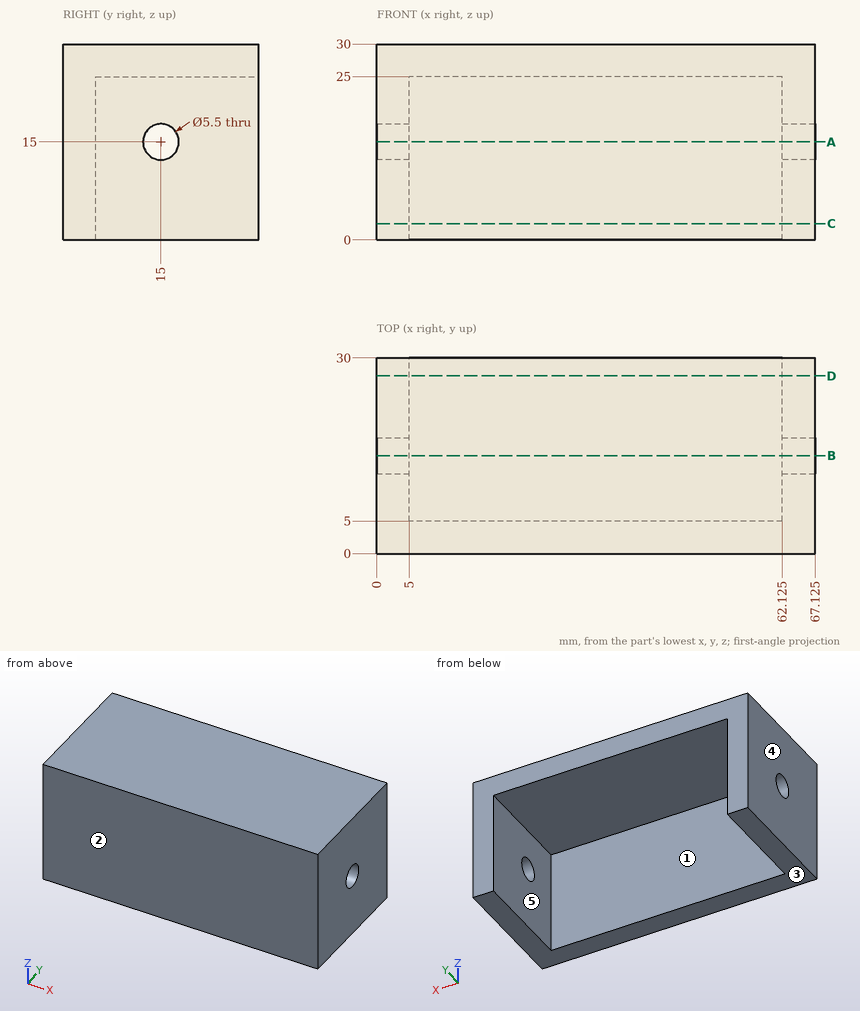
Design review of the part shown in the three views and the two pictorial views. Dimensions are in mm from the part's minimum x, y and z. A direction names the side the tool comes from. Round coordinates to 2 decimals unless told otherwise and drop trailing zeros. Order: outer loops, then holes, each group sorted by start corner. A loop starts at its lowest first (then second) coordinate and runs counter-clockwise, first axis right, second up.
(1) Mouldability with a two-part tool opening along X and no side actions: class the marked faces 3, 4 and 5 as released by +X, released by -X, zero draft, split by the parting line, or undercut.
Working result:
face 3: zero draft
face 4: released by -X
face 5: undercut
(2) For P1, Ø3, axis at x = 58.5, z = 15, coming from the +Y side; P2, Ø12.5, axis at x = 46.5, y = 23, coming from the -Z side, all flat-tipped, find the tip position at first contact; note any pin that passes through.
Working result:
P1: stops at y = 5
P2: stops at z = 25
(3) Take a section at C-C, the plane z = 2.5. State the section outline as (x, y) points (3 decimals).
Working result:
outline: (0, 0) - (67.125, 0) - (67.125, 30) - (62.125, 30) - (62.125, 5) - (5, 5) - (5, 30) - (0, 30) - close
(4) Take a section at A-A, the plane z = 15. State the section outline as (x, y) points (3 decimals).
Working result:
outline: (0, 0) - (67.125, 0) - (67.125, 12.25) - (62.125, 12.25) - (62.125, 5) - (5, 5) - (5, 12.25) - (0, 12.25) - close; (0, 17.75) - (5, 17.75) - (5, 30) - (0, 30) - close; (62.125, 17.75) - (67.125, 17.75) - (67.125, 30) - (62.125, 30) - close
(5) Take a section at D-D, the plane y = 27.25. State the section outline as (x, z) points (3 decimals), plus the area to 3 significant figures.
Working result:
outline: (0, 0) - (5, 0) - (5, 25) - (62.125, 25) - (62.125, 0) - (67.125, 0) - (67.125, 30) - (0, 30) - close
area: 586 mm2
(6) Wall thickness on L1, parallel to X at y = 27.75, z = 14 (3 decimals); L2, parallel to Y at x = 1.7, z = 15; L3, parallel to Z at x = 57.5, y = 7.5: over which ranges is each line inside the solid? List them lowest first.
Working result:
L1: x = 0 to 5, 62.125 to 67.125
L2: y = 0 to 12.25, 17.75 to 30
L3: z = 25 to 30
(7) Take a section at B-B, the plane y = 15. State the section outline as (x, z) points (3 decimals).
Working result:
outline: (0, 0) - (5, 0) - (5, 12.25) - (0, 12.25) - close; (0, 17.75) - (5, 17.75) - (5, 25) - (62.125, 25) - (62.125, 17.75) - (67.125, 17.75) - (67.125, 30) - (0, 30) - close; (62.125, 0) - (67.125, 0) - (67.125, 12.25) - (62.125, 12.25) - close
(8) Tool access review of the marked faces 1 and 2: name each direction out of +Z, -Z, +X, -X, +Y, -Y from which nothing blocks a thin tool from reaching the whole face with its end or side.
Working result:
face 1: -Z, +Y
face 2: +Z, -Z, +X, -X, -Y
